Check sheet for the drawn part. Datum: minimum x, y, z corner. Units: mm. A direction names the side the tool comes from. Round coordinates to 2 decimals unless told otherwise and drop trailing zeros. Loops run counter-clockwise (first coordinate to the right, second up) from the corner with the lowest first, then second, coordinate; pieces in that order, holes last.
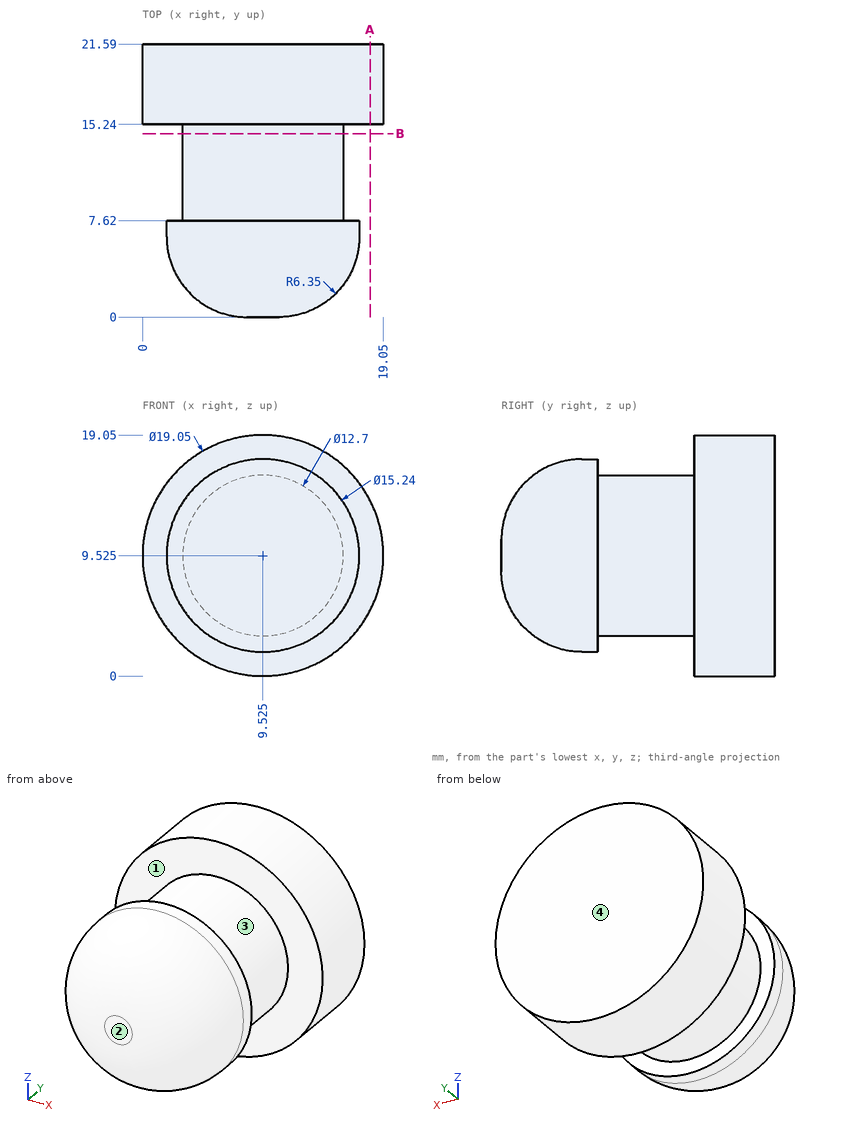
1) Gauge pin test, flat ends, axial feed: pin 1 (3 mm diameter, centred on x = 15, y = 7.5, fed in from +Z); pin 2 (5.5 mm diameter, centred on x = 13, z = 7, fed in from -Y); pin 3 (1.5 mm diameter, centred on x = 10, y = 6.5, fed in from -Z) (3 decimals). Record the tip position at first contact, or that the pin passes through.
Report:
pin 1: stops at z = 16.03
pin 2: stops at y = 0.01
pin 3: stops at z = 1.905
2) Sectioned sample at A-A, the plane x = 18. Record the cut outline in (y, z), then the cut area to 3 significant figures.
Report:
outline: (15.24, 5.18) - (21.59, 5.18) - (21.59, 13.87) - (15.24, 13.87) - close
area: 55.2 mm2
3) Sectioned sample at B-B, the plane y = 14.5. Record the cut outline in (x, z) (3 decimals).
Report:
outline: circle Ø12.7 at (9.525, 9.525)
4) Scan lines: line 1 along Y through (x, z) = (17, 7); line 2 along X through (y, z) = (8.25, 9.75); line 3 along X through (y, z) = (3.75, 6.5). Record each from-to range of solid material in increasing order.
Report:
line 1: y = 15.24 to 21.59
line 2: x = 3.18 to 15.87
line 3: x = 3.14 to 15.91
5) Mould release check, pull along Z, two halves, no side actions. Record for the marked faces 3 and 4: +Z half, -Z half, draft (parallel to the pull), parting line (faces both ways), or undercut.
Report:
face 3: parting line
face 4: draft
6) Access from +Z, -Z, +X, -X, +Y, -Y to the whole of each face (thin tool, end or side, straight path). Record for the marked faces 1 and 2.
Report:
face 1: none
face 2: +Z, -Z, +X, -X, -Y
